from build123d import *

# Parameters (mm, degrees)
F1_DEPTH  = 2
F2_W      = 16
F2_H      = 12
F3_DEPTH  = 11
F4_W      = 14
F4_H      = 9
F5_DEPTH  = 11
F6_W      = 16
F6_H      = 2.5
F7_DEPTH  = 9
F8_W      = 21
F8_H      = 2.5
F9_DEPTH  = 4
F10_W     = 21
F10_H     = 2.5
F10_W_2   = 26
F11_DEPTH = 4
F13_DEPTH = 12
F14_R     = 3
F15_DEPTH = 12
F17_DEPTH = 12
F18_SIZE2 = 2.99999
F18_SIZE  = 2.99999
F19_SIZE2 = 1
F19_SIZE  = 1
F20_R     = 1.5
F21_DEPTH = 2


# Not quite as in the source:
# - a fillet or chamfer is up to 0.001 mm smaller than in the source, because OpenCascade refuses the exact size


with BuildPart() as f1:
    # F0 (on Top) → F1 (new body)
    with BuildSketch(Plane.XY):
        Polygon((3, 11), (3, 0), (69, 0), (69, 53), (3, 53), (3, 51), (0, 51), (0, 11), align=None)
    extrude(amount=F1_DEPTH)

    # F2 (on face) → F3 (join)
    with BuildSketch(Plane.XY.offset(2)):
        with Locations((69, 15)):
            Rectangle(F2_W, F2_H)
    extrude(amount=F3_DEPTH)

    # F4 (on face) → F5 (join)
    with BuildSketch(Plane.XY.offset(2)):
        with Locations((66, 44.5)):
            Rectangle(F4_W, F4_H)
    extrude(amount=F5_DEPTH)

    # F6 (on face) → F7 (join)
    with BuildSketch(Plane.XY.offset(2)):
        with Locations((12, 50.25)):
            Rectangle(F6_W, F6_H)
    extrude(amount=F7_DEPTH)

    # F8 (on face) → F9 (join)
    with BuildSketch(Plane.XY.offset(2)):
        with Locations((32.5, 50.75)):
            Rectangle(F8_W, F8_H)
    extrude(amount=F9_DEPTH)

    # F10 (on face) → F11 (join)
    with BuildSketch(Plane.XY.offset(2)):
        with Locations((14.5, 2.75)):
            Rectangle(F10_W, F10_H)
        with Locations((39, 2.75)):
            Rectangle(F10_W_2, F10_H)
    extrude(amount=F11_DEPTH)

    # F12 (on face) → F13 (cut)
    with BuildSketch(Plane(origin=(59, 0, 0), x_dir=(0, -1, 0), z_dir=(-1, 0, 0))):
        with BuildLine():
            ThreePointArc((-49, 8.5), (-44.5, 13), (-40, 8.5))
            Line((-40, 8.5), (-38.6329554021, 9.580289945))
            Line((-38.6329554021, 9.580289945), (-38.187738508, 14.0570942312))
            Line((-38.187738508, 14.0570942312), (-42.2688946128, 14.7991068661))
            Line((-42.2688946128, 14.7991068661), (-51.2474328279, 13.8839585707))
            Line((-51.2474328279, 13.8839585707), (-49, 8.5))
        make_face()
        Polygon((-40, 13), (-40, 8.5), (-38.6329554021, 9.580289945), (-38.187738508, 14.0570942312), (-42.2688946128, 14.7991068661), (-51.2474328279, 13.8839585707), (-49, 8.5), (-49, 13), (-44.5, 13), align=None)
    extrude(amount=-F13_DEPTH, mode=Mode.SUBTRACT)

    # F14 (on face) → F15 (cut)
    with BuildSketch(Plane.YZ.offset(73)):
        with Locations((44.5, 8.5)):
            Circle(F14_R)
    extrude(amount=-F15_DEPTH, mode=Mode.SUBTRACT)

    # F16 (on face) → F17 (cut)
    with BuildSketch(Plane.YZ.offset(77)):
        Polygon((18, 12), (12, 12), (10, 10), (10, 3), (20, 3), (20, 10), align=None)
    extrude(amount=-F17_DEPTH, mode=Mode.SUBTRACT)

    # F18 (size 3 and 3 in the source; OpenCascade refuses exactly that, so slightly less here)
    f18_edges = [f1.edges().sort_by_distance(p)[0] for p in [
        (0, 51, 1),
        (0, 11, 1),
    ]]
    chamfer(f18_edges, length=F18_SIZE, length2=F18_SIZE2)

    # F19
    f19_edges = [f1.edges().sort_by_distance(p)[0] for p in [
        (3, 0, 1),
        (69, 0, 1),
        (69, 53, 1),
        (3, 53, 1),
    ]]
    chamfer(f19_edges, length=F19_SIZE, length2=F19_SIZE2)

    # F20 (on face) → F21 (cut)
    with BuildSketch(Plane.XY.offset(2)):
        with Locations((3, 16)):
            Circle(F20_R)
        with Locations((3, 44)):
            Circle(F20_R)
    extrude(amount=-F21_DEPTH, mode=Mode.SUBTRACT)


solid = f1.part
The listing builds one solid part. Answer for the finished solid, in the listing's coordinates (mm). A direction names the side the tool comes from. Give positions to 0.01 mm unless a question says otherwise; leave off trailing zeros. Write each loop counter-clockwise with the first axis right and the second up, starting at its lowest first coordinate (ties: lowest second). Pieces come first, ordered by that corner, then holes. Notation, with made-up numbers: (28, 43) - (46, 43) arc R22 cw to (46, 60) - close; hole circle Ø2 at (10, 75.25). An arc over 180 degrees is marked (long way). Use a Markdown table: item, result.
1. A tool of negligible diameter and unlimited length cuts with its end or side. For faces 1 (the flat face through (69, 21, 7)), 2 (the flat face through (22, 51, 4)), 3 (the flat face through (71, 10, 7)), from which of +Z, -Z, +X, -X, +Y, -Y can it reach the whole face along a straight path? Write none if from no direction.
Values follow:
| item | result |
|---|---|
| face 1 | +Z, +X, -X |
| face 2 | +Z, +Y |
| face 3 | +X |
2. For a pull along Y with two mould halves and no side action, classify faces 4 (the cylindrical face through (2.675, 42.536, 1.014)), 5 (the flat face through (32, 52, 4)), 6 (the flat face through (73, 44, 5)) as released by +Y, released by -Y, zero draft, split by the parting line, or undercut.
Values follow:
| item | result |
|---|---|
| face 4 | undercut |
| face 5 | released by +Y |
| face 6 | zero draft |
3. Section C-C on z = 7 is taken. Write down the section's boundary in (x, y).
Values follow:
| item | result |
|---|---|
| outline | (4, 49) - (20, 49) - (20, 51.5) - (4, 51.5) - close; (59, 40) - (73, 40) - (73, 41.9) - (61, 41.9) - (61, 47.1) - (73, 47.1) - (73, 49) - (59, 49) - close; (61, 9) - (77, 9) - (77, 10) - (65, 10) - (65, 20) - (77, 20) - (77, 21) - (61, 21) - close |
4. Section D-D on y = 32.5 is taken. Write down the section's boundary in (x, z).
Values follow:
| item | result |
|---|---|
| outline | (0, 0) - (69, 0) - (69, 2) - (0, 2) - close |
5. Each of these flat-tipped pins is pushed along its axis until it touches: P1, Ø5.5, axis at x = 72, z = 9.5, coming from the +Y side; P2, Ø16, axis at x = 47.5, y = 20.5, coming from the +Z side; P3, Ø1, axis at x = 66.5, z = 8, coming from the -Y side. Where does it stop, or does it pass through?
Values follow:
| item | result |
|---|---|
| P1 | stops at y = 49 |
| P2 | stops at z = 2 |
| P3 | stops at y = 9 |
6. Find the intervals of material crossed by probe 1 along Z at (x, y) = (33.5, 34); probe 2 along Z at (x, y) = (12, 49.5); probe 3 along X at (y, z) = (18, 8.5), in increasing order. Write a range as from..to.
Values follow:
| item | result |
|---|---|
| probe 1 | z = 0..2 |
| probe 2 | z = 0..11 |
| probe 3 | x = 61..65 |
7. Section A-A on y = 16 is taken. Write down the section's boundary in (x, z), plus the area to 3 significant figures.
Values follow:
| item | result |
|---|---|
| outline | (0, 0) - (1.5, 0) - (1.5, 2) - (0, 2) - close; (4.5, 0) - (69, 0) - (69, 2) - (77, 2) - (77, 3) - (65, 3) - (65, 12) - (77, 12) - (77, 13) - (61, 13) - (61, 2) - (4.5, 2) - close |
| area | 200 mm² |
8. Section B-B on x = 37 is taken. Write down the section's boundary in (y, z), plus the area to 3 significant figures.
Values follow:
| item | result |
|---|---|
| outline | (0, 0) - (53, 0) - (53, 2) - (52, 2) - (52, 6) - (49.5, 6) - (49.5, 2) - (4, 2) - (4, 6) - (1.5, 6) - (1.5, 2) - (0, 2) - close |
| area | 126 mm² |
